Design review of the part built by this model. Coordinates are the model's own, in mm. Coordinates: 2 decimals unless noted, no trailing zeros. Write each loop counter-clockwise with the first axis right and the second up, starting at its lowest first coordinate (ties: lowest second). Pieces come first, ordered by that corner, then holes.
Q1. Take a section at C-C, the plane x = -36. Write out the cut boundary in (y, z), plus the area to 3 significant figures.
Q2. Take a section at B-B, the plane y = 7.5. State how many separate pieces and enclosed holes the cut face has, plus the area to 3 significant figures.
Q3. Take a section at A-A, the plane x = -11. Write out the cut boundary in (y, z), plus the area to 3 significant figures.
Q4. For L1, parallel to Y at x = -10.5, z = 4.1; L2, parallel to Y at x = -37, z = 1.05; L3, parallel to Y at x = -4.5, z = 3.55, list the stretches that pass through material, from the lowest coordinate up.
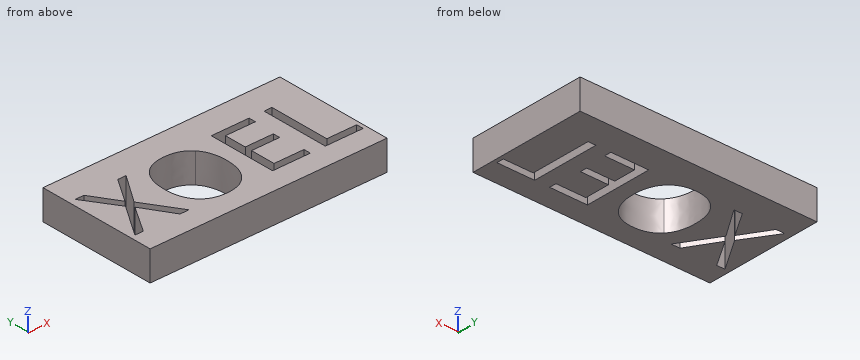
from build123d import *

# Parameters (mm, degrees)
F0_W     = 7.3027783253
F0_H     = 2
F1_DEPTH = 5


with BuildPart() as f1:
    # F0 (on Top) → F1 (new body)
    with BuildSketch(Plane.XY):
        Polygon((-6.9230771488, 20), (-32.6972216747, 20), (-32.6972216747, 18), (-40, 18), (-40, 0), (0, 0), (0, 20), align=None)
        Polygon((-33.8621847978, 9.7746401855), (-30.0435746334, 3.750000149), (-31.5534906525, 3.750000149), (-34.6284108374, 8.7805495395), (-37.7584191689, 3.750000149), (-39.1681749214, 3.750000149), (-35.364588797, 9.7295680656), (-38.9102622349, 15.1908066024), (-37.4379063158, 15.1908066024), (-34.5983627574, 10.6585545384), (-31.7337791324, 15.1908066024), (-30.3190153665, 15.1908066024), align=None, mode=Mode.SUBTRACT)
        with BuildLine():
            add(Edge.make_bspline(
                [(-19.8622835325, 13.8060909166), (-18.4775678467, 12.2410867508), (-18.4775678467, 9.486679419)],
                knots=[0, 0, 0, 1, 1, 1], degree=2))
            add(Edge.make_bspline(
                [(-18.4775678467, 9.486679419), (-18.4775678467, 6.7397841073), (-19.8672915459, 5.1660159182)],
                knots=[0, 0, 0, 1, 1, 1], degree=2))
            add(Edge.make_bspline(
                [(-19.8672915459, 5.1660159182), (-21.2570152451, 3.5922477291), (-23.7284698237, 3.5922477291)],
                knots=[0, 0, 0, 1, 1, 1], degree=2))
            add(Edge.make_bspline(
                [(-23.7284698237, 3.5922477291), (-26.2550125489, 3.5922477291), (-27.6284602047, 5.1384718449)],
                knots=[0, 0, 0, 1, 1, 1], degree=2))
            add(Edge.make_bspline(
                [(-27.6284602047, 5.1384718449), (-29.0019078606, 6.6846959607), (-29.0019078606, 9.501703459)],
                knots=[0, 0, 0, 1, 1, 1], degree=2))
            add(Edge.make_bspline(
                [(-29.0019078606, 9.501703459), (-29.0019078606, 12.2961748974), (-27.6247041947, 13.8336349899)],
                knots=[0, 0, 0, 1, 1, 1], degree=2))
            add(Edge.make_bspline(
                [(-27.6247041947, 13.8336349899), (-26.2475005289, 15.3710950823), (-23.7134457837, 15.3710950823)],
                knots=[0, 0, 0, 1, 1, 1], degree=2))
            add(Edge.make_bspline(
                [(-23.7134457837, 15.3710950823), (-21.2469992184, 15.3710950823), (-19.8622835325, 13.8060909166)],
                knots=[0, 0, 0, 1, 1, 1], degree=2))
        make_face(mode=Mode.SUBTRACT)
        Polygon((-9.5507840851, 4.939403315), (-9.5507840851, 3.750000149), (-15.9284890615, 3.750000149), (-15.9284890615, 15.1908066024), (-9.5507840851, 15.1908066024), (-9.5507840851, 14.0089154564), (-14.5988615222, 14.0089154564), (-14.5988615222, 10.3230176452), (-9.8562728983, 10.3230176452), (-9.8562728983, 9.1486385192), (-14.5988615222, 9.1486385192), (-14.5988615222, 4.939403315), align=None, mode=Mode.SUBTRACT)
        Polygon((-0.6390243636, 3.750000149), (-7.0167293399, 3.750000149), (-7.0167293399, 15.1908066024), (-5.6871018007, 15.1908066024), (-5.6871018007, 4.954427355), (-0.6390243636, 4.954427355), align=None, mode=Mode.SUBTRACT)
        with BuildLine():
            ThreePointArc((-4.5192325674, 17.596155405), (-8.6228519812, 15.8963805958), (-6.9230771488, 20))
            ThreePointArc((-6.9230771488, 20), (-5.2233023436, 19.2959302143), (-4.5192325674, 17.596155405))
        make_face(mode=Mode.SUBTRACT)
        with BuildLine():
            ThreePointArc((-4.5192325674, 17.596155405), (-5.2233023436, 19.2959302143), (-6.9230771488, 20))
            ThreePointArc((-6.9230771488, 20), (-8.6228519812, 15.8963805958), (-4.5192325674, 17.596155405))
        make_face()
        with Locations((-36.3486108374, 19)):
            Rectangle(F0_W, F0_H)
    extrude(amount=F1_DEPTH)


solid = f1.part
Responses:
1. outline: (0, 0) - (6.58, 0) - (6.58, 5) - (0, 5) - close; (8.73, 0) - (10.71, 0) - (10.71, 5) - (8.73, 5) - close; (12.9, 0) - (20, 0) - (20, 5) - (12.9, 5) - close
1. area: 78.3 mm2
2. separate pieces: 6
2. enclosed holes: 0
2. area: 122 mm2
3. outline: (0, 0) - (3.75, 0) - (3.75, 5) - (0, 5) - close; (4.94, 0) - (9.15, 0) - (9.15, 5) - (4.94, 5) - close; (10.32, 0) - (14.01, 0) - (14.01, 5) - (10.32, 5) - close; (15.19, 0) - (20, 0) - (20, 5) - (15.19, 5) - close
3. area: 82.3 mm2
4. L1: y = 0 to 3.75, 4.94 to 9.15, 10.32 to 14.01, 15.19 to 20
4. L2: y = 0 to 4.97, 7.16 to 12.25, 14.49 to 20
4. L3: y = 0 to 3.75, 4.95 to 20
